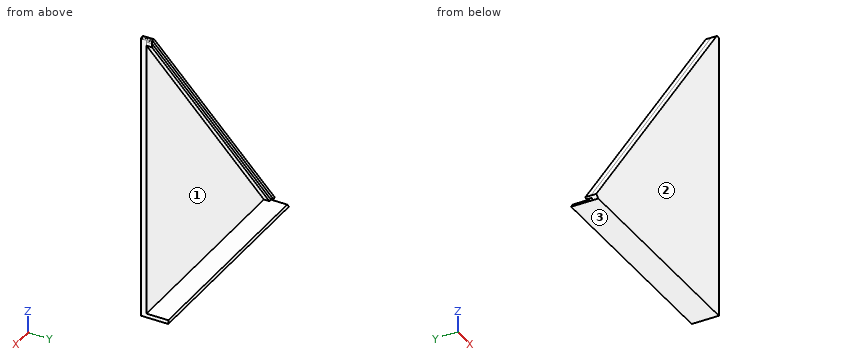
Autodesk Inventor part; units mm, degrees
ref_plane "YZ Plane" through (0, 0, 0) normal (1, 0, 0) x (0, 1, 0)
ref_plane "XZ Plane" through (0, 0, 0) normal (0, 1, 0) x (-1, 0, 0)
ref_plane "XY Plane" through (0, 0, 0) normal (0, 0, 1) x (1, 0, 0)
sketch "Skizze1" plane through (0, 0, 0) normal (0, 1, 0) x (-1, 0, 0)
  line L0 (0, 0) -> (198.599, 0)
  line L1 (198.599, 0) -> (0, 263.5497)
  line L2 (0, 263.5497) -> (0, 0)
  line L3 (-198.599, 0) -> (0, -263.5497)
  line L4 (0, 0) -> (-198.599, 0)
  line L5 (-198.599, 0) -> (0, -263.5497)
  line L6 (0, -263.5497) -> (-3.3543, -266.0773)
  line L7 (-3.3543, -266.0773) -> (-201.9532, -2.5276)
  line L8 (-201.9532, -2.5276) -> (-198.599, 0)
  line L9 (-195.878, -3.6109) -> (0, -3.6109)
  line L10 (0, -263.5497) -> (0, 0)
  line L11 (0, -3.6109) -> (0, 0)
  line L12 (-1.6771, -264.8135) -> (-200.2761, -1.2638)
  line L13 (-195.878, -3.6109) -> (-198.599, 0)
  line L14 (0, 0) -> (-198.599, 0)
  line L15 (-1.6771, -264.8135) -> (-3.3543, -266.0773)
  line L16 (0, 263.5497) -> (1.6771, 264.8135)
  line L17 (1.6771, 264.8135) -> (200.2761, 1.2638)
  line L18 (200.2761, 1.2638) -> (198.599, 0)
  line L19 (200.2761, 1.2638) -> (201.9532, 2.5276)
  line L20 (201.9532, 2.5276) -> (3.9544, 265.281)
  line L21 (3.3543, 266.0773) -> (1.6771, 264.8135)
  line L22 (2.3571, 266.0773) -> (1, 266.0773)
  line L23 (0, 265.0773) -> (0, 263.5497)
  arc A0 (3.9544, 265.281) -> (2.3571, 266.0773) centre (2.3571, 264.0773) ccw
  arc A1 (1, 266.0773) -> (0, 265.0773) centre (1, 265.0773) ccw
  point P0 (3.1416, 265.9171)
  dimension "d0" = 37
  dimension "d1" = 330
  dimension "d7" = 4.2
  dimension "d8" = 2.1
  dimension "d9" = 2.1
  dimension "d11" = 2
  dimension "d12" = 1
extrude "Extrusion1" add sketch "Skizze1" along normal blind 5 contours L2 L1 L0 | L1 L16 L17 L18 | L23 A1 L22 A0 L21 L16 | L17 L21 A0 L20 L19
sketch "Skizze2" plane through (0, 5, 0) normal (0, 1, 0) x (1, 0, 0)
  line L0 (-198.599, 0) -> (0, -263.5497)
  line L1 (0, 0) -> (-198.599, 0)
  line L2 (-198.599, 0) -> (0, -263.5497)
  line L3 (0, -263.5497) -> (-3.1416, -265.9171)
  line L4 (-3.3543, -266.0773) -> (-201.9532, -2.5276)
  line L5 (-201.9532, -2.5276) -> (-198.599, 0)
  line L6 (-195.878, -3.6109) -> (0, -3.6109)
  line L7 (0, -263.5497) -> (0, 0)
  line L8 (0, -3.6109) -> (0, 0)
  line L9 (-1.6771, -264.8135) -> (-200.2761, -1.2638)
  line L10 (-195.878, -3.6109) -> (-198.599, 0)
  line L11 (0, 0) -> (-198.599, 0)
  line L12 (-1.6771, -264.8135) -> (-3.3543, -266.0773)
  line L13 (-193.2485, -3.6109) -> (0, -260.0603)
  line L14 (0, -260.0603) -> (0, -263.5497)
  line L15 (0, -265.0773) -> (0, 0)
  line L16 (0, 0) -> (-198.599, 0)
  line L17 (-198.599, 0) -> (-201.9532, -2.5276)
  line L18 (-201.9532, -2.5276) -> (-3.9544, -265.281)
  arc A0 (-3.9544, -265.281) -> (-2.3571, -266.0773) centre (-2.3571, -264.0773) ccw
  line L19 (-2.3571, -266.0773) -> (-1, -266.0773)
  arc A1 (-1, -266.0773) -> (0, -265.0773) centre (-1, -265.0773) ccw
  line L20 (-3.1416, -265.9171) -> (-3.3543, -266.0773)
  point P0 (-3.9544, -265.281)
  dimension "d4" = 4.2
  dimension "d10" = 2.1
extrude "Extrusion2" add sketch "Skizze2" along normal blind 5 contours L6 L13 L7 L0 | L9 L3 A0 L4 L5 | L15 A1 L19 A0 L3
extrude "Extrusion3" add sketch "Skizze2" along normal blind 20 contours L1 L7 L6 L0
properties part number "SolarMountLeft"
Model file for the job. Use its own axes, mm. Face numbers are marked on the shaded views. Round coordinates to 2 decimals unless told otherwise and drop trailing zeros. Write each loop counter-clockwise with the first axis right and the second up, starting at its lowest first coordinate (ties: lowest second). Pieces come first, ordered by that corner, then holes. Notation, with made-up numbers: (19.25, 47) - (34.25, 47) arc R14 ccw to (34.25, 59) - close; hole circle Ø7 at (41, -39.5). An arc over 180 degrees is marked (long way). Use CSV: the item, a comma, the result in double quotes. Start each with the question number.
Item 1: Drill centre lines: L1, parallel to Z at x = -10.5, y = 5.25; L2, parallel to Y at x = -53.5, z = 177; L3, parallel to Z at x = -7.5, y = 8.25. Where is each one in solid material? Low to high. Write a range as [from, to].
Item 2: Band-saw the part on C-C (y = 16.5). Write the cut outline in (x, z).
Item 3: Two-plate mould, pull along Z, no slides. Class the marked faces 1, 2 and 3: released by +Z, released by -Z, zero draft, split by the parting line, or undercut.
Item 4: Band-saw the part on B-B (z = 59). Write the cut outline in (x, y).
Item 5: Pin check, flat tips, straight feed: P1, Ø10, axis at x = -163, y = 10.5, coming from the +Z side; P2, Ø12, axis at y = 4.5, z = 176.5, coming from the -X side. Stop position of each tip, or through.
Item 6: Band-saw the part on D-D (x = -96). Write the cut outline in (y, z), and give its area (3 significant figures).
Item 7: Band-saw the part on A-A (x = -125). Write the cut outline in (y, z).
Checked values:
1,L1,"z = [0, 3.61], [246.13, 249.62], [253.11, 256.59]"
1,L2,"y = [0, 5]"
1,L3,"z = [0, 3.61], [250.11, 253.6], [257.09, 260.58]"
2,outline,"(-198.6, 0) - (0, 0) - (0, 3.61) - (-195.88, 3.61) - close"
3,face 1,"undercut"
3,face 2,"zero draft"
3,face 3,"released by -Z"
4,outline,"(-159.4, 0) - (0, 0) - (0, 5) - (-151.51, 5) - (-151.51, 10) - (-154.14, 10) - (-154.14, 5) - (-156.77, 5) - (-156.77, 10) - (-159.4, 10) - close"
5,P1,"stops at z = 60.82"
5,P2,"stops at x = -75.38"
6,outline,"(0, 0) - (25, 0) - (25, 3.61) - (5, 3.61) - (5, 132.66) - (10, 132.66) - (10, 136.15) - (5, 136.15) - (5, 139.64) - (10, 139.64) - (10, 143.13) - (0, 143.13) - close"
6,area,"823 mm²"
7,outline,"(0, 0) - (25, 0) - (25, 3.61) - (5, 3.61) - (5, 94.18) - (10, 94.18) - (10, 97.67) - (5, 97.67) - (5, 101.16) - (10, 101.16) - (10, 104.65) - (0, 104.65) - close"
